```python
from build123d import *

# Parameters (mm, degrees)
SKETCH1_R           = 1.5
SKETCH1_R_2         = 2.5
BOSS_EXTRUDE1_DEPTH = 10
SKETCH4_W           = 110
SKETCH4_H           = 10
BOSS_EXTRUDE2_DEPTH = 55
SKETCH6_R           = 3
SKETCH6_R_2         = 11
CUT_EXTRUDE1_DEPTH  = 246.089779469
FILLET1_R           = 5
FILLET2_R           = 15
CUT_EXTRUDE2_DEPTH  = 5


with BuildPart() as part:
    # Sketch1 → Boss-Extrude1 (new body)
    with BuildSketch(Plane.XY):
        Polygon((20, 0), (90, 0), (110, 0), (110, 200), (110, 212), (90, 212), (90, 200), (20, 200), (20, 212), (0, 212), (0, 200), (0, 0), align=None)
        with Locations((100, 10)):
            Circle(SKETCH1_R, mode=Mode.SUBTRACT)
        with Locations((80, 10)):
            Circle(SKETCH1_R, mode=Mode.SUBTRACT)
        with Locations(Location((100, 30, 0), (0, 0, 180))):
            Circle(SKETCH1_R, mode=Mode.SUBTRACT)
        with Locations(Location((80, 30, 0), (0, 0, 180))):
            Circle(SKETCH1_R, mode=Mode.SUBTRACT)
        with Locations(Location((30, 10, 0), (0, 0, 180))):
            Circle(SKETCH1_R, mode=Mode.SUBTRACT)
        with Locations(Location((10, 10, 0), (0, 0, 180))):
            Circle(SKETCH1_R, mode=Mode.SUBTRACT)
        with Locations((10, 30)):
            Circle(SKETCH1_R, mode=Mode.SUBTRACT)
        with Locations((30, 30)):
            Circle(SKETCH1_R, mode=Mode.SUBTRACT)
        with Locations(Location((100, 107.5, 0), (0, 0, 180))):
            Circle(SKETCH1_R, mode=Mode.SUBTRACT)
        with Locations((100, 87.5)):
            Circle(SKETCH1_R, mode=Mode.SUBTRACT)
        with Locations((80, 87.5)):
            Circle(SKETCH1_R, mode=Mode.SUBTRACT)
        with Locations(Location((80, 107.5, 0), (0, 0, 180))):
            Circle(SKETCH1_R, mode=Mode.SUBTRACT)
        with Locations((30, 107.5)):
            Circle(SKETCH1_R, mode=Mode.SUBTRACT)
        with Locations((10, 107.5)):
            Circle(SKETCH1_R, mode=Mode.SUBTRACT)
        with Locations(Location((30, 87.5, 0), (0, 0, 180))):
            Circle(SKETCH1_R, mode=Mode.SUBTRACT)
        with Locations(Location((10, 87.5, 0), (0, 0, 180))):
            Circle(SKETCH1_R, mode=Mode.SUBTRACT)
        with Locations((48.5, 68.75)):
            Circle(SKETCH1_R_2, mode=Mode.SUBTRACT)
        with Locations((48.5, 48.75)):
            Circle(SKETCH1_R_2, mode=Mode.SUBTRACT)
    extrude(amount=BOSS_EXTRUDE1_DEPTH)

    # Sketch4 → Boss-Extrude2 (add)
    with BuildSketch(Plane(origin=(0, 0, 0), x_dir=(-1, 0, 0), z_dir=(0, 0, -1))):
        with Locations((-55, -5)):
            Rectangle(SKETCH4_W, SKETCH4_H)
    extrude(amount=-BOSS_EXTRUDE2_DEPTH)

    # Sketch6 → Cut-Extrude1 (cut, through all)
    with BuildSketch(Plane(origin=(0, 0, 0), x_dir=(1, 0, 0), z_dir=(0, 1, 0))):
        with Locations(Location((95, -40, 0), (0, 0, 180))):
            Circle(SKETCH6_R)
        with Locations(Location((15, -40, 0), (0, 0, 180))):
            Circle(SKETCH6_R)
        with Locations(Location((55, -27.5, 0), (0, 0, 180))):
            Circle(SKETCH6_R_2)
    extrude(amount=-CUT_EXTRUDE1_DEPTH, mode=Mode.SUBTRACT)

    # Fillet1
    fillet1_edges = [part.edges().sort_by_distance(p)[0] for p in [
        (55, 0, 10),
    ]]
    fillet(fillet1_edges, radius=FILLET1_R)

    # Fillet2
    fillet2_edges = [part.edges().sort_by_distance(p)[0] for p in [
        (0, -5, 55),
        (110, -5, 55),
    ]]
    fillet(fillet2_edges, radius=FILLET2_R)

    # Sketch7 → Cut-Extrude2 (cut)
    with BuildSketch(Plane.XY.offset(10)):
        Polygon((46.190598923, 72.75), (43.881197846, 68.75), (46.190598923, 64.75), (50.809401077, 64.75), (53.118802154, 68.75), (50.809401077, 72.75), align=None)
        Polygon((50.809401077, 52.75), (46.190598923, 52.75), (43.881197846, 48.75), (46.190598923, 44.75), (50.809401077, 44.75), (53.118802154, 48.75), align=None)
    extrude(amount=-CUT_EXTRUDE2_DEPTH, mode=Mode.SUBTRACT)


solid = part.part
```
Source: CAD feature listing. Evaluate the final solid. Frame: model axes, mm. A direction names the side the tool comes from. Coordinates: 2 decimals unless noted, no trailing zeros. Loops run counter-clockwise (first coordinate to the right, second up) from the corner with the lowest first, then second, coordinate; pieces in that order, holes last. Notation, with made-up numbers: M 54.5,48.5 L 98.5,48.5 A30 cw 98.5,81.5 Z; hole C 42,42 d6. An arc over 180 degrees is marked long. Put each result on its own line as item: value. Start each with the question number.
1) Ray query, L1, parallel to Y at x = 30, z = 3; L2, parallel to Y at x = 100, z = 3; L3, parallel to Y at x = 48.5, z = 1.2. Return the intervals inside material, ascending. Write a range as from..to.
2) Reachability of faces 1 (the face through (90, 206, 5)), 2 (the face through (50.5, 67, 5)), 3 (the face through (0, 92.3, 9.5)), 4 (the face through (54, 110, 10)) from +Z, -Z, +X, -X, +Y, -Y: full face, straight path, thin tool, end or side. Return the list, or none.
3) Cut plane D-D on y = 56. Return the cut outline in (x, z), then the cut area to 3 significant figures.
4) Cut plane C-C on x = 87.5. Return the cut outline in (y, z).
5) Pull-direction query (X, two-part tool) for faces 5 (the face through (51.98, 70.72, 7.54)), 6 (the face through (110, 92.3, 9.5)), 7 (the face through (100, 212, 5)); classes: pulls with the +X half, pulls with the -X half, needs draft (parallel to the pull), parting line crosses it, or undercut.
6) Contact query for flat-ended pins moving along their axis: pin 1 Ø3.5 at (x, z) = (49.5, 8) entering from +Y; pin 2 Ø2.5 at (x, y) = (80, 10) entering from -Z; pin 3 Ø6 at (x, y) = (48.5, 48.75) entering from +Z; pin 4 Ø6 at (x, y) = (89, 81) entering from +Z. Output: stop coordinate, or through.
7) Cut plane A-A on z = 24. Return the cut outline in (x, y).
8) Cut plane B-B on x = 55.5. Return the cut outline in (y, z).
The answers:
1. L1: y = -10..8.5, 11.5..28.5, 31.5..86, 89..106, 109..200
1. L2: y = -10..8.5, 11.5..28.5, 31.5..86, 89..106, 109..212
1. L3: y = -10..46.25, 51.25..66.25, 71.25..200
2. face 1: +Z, -Z, +Y
2. face 2: +Z
2. face 3: +Z, -Z, -X, +Y, -Y
2. face 4: +Z, +X, -X, +Y
3. outline: M 0,0 L 110,0 L 110,10 L 0,10 Z
3. area: 1,100 mm²
4. outline: M -10,0 L 200,0 L 200,10 L 5,10 A5 cw 0,15 L 0,55 L -10,55 Z
5. face 5: undercut
5. face 6: pulls with the +X half
5. face 7: needs draft
6. pin 1: stops at y = 200
6. pin 2: passes through
6. pin 3: stops at z = 5
6. pin 4: stops at z = 10
7. outline: M 0,-10 L 44.57,-10 L 44.57,0 L 0,0 Z; M 65.43,-10 L 110,-10 L 110,0 L 65.43,0 Z
8. outline: M -10,0 L 200,0 L 200,10 L 5,10 A5 cw 0,15 L 0,16.51 L -10,16.51 Z; M -10,38.49 L 0,38.49 L 0,55 L -10,55 Z
